Part model, mm, in its own coordinate system. Face numbers are marked on the shaded views. Give positions to 0.01 mm unless a question says otherwise; leave off trailing zeros. Order: outer loops, then holes, each group sorted by start corner. A loop starts at its lowest first (then second) coordinate and runs counter-clockwise, first axis right, second up. Notation, with made-up numbers: M 43,24 L 94,24 A33 cw 94,62 Z; hole C 55.5,49 d3. An arc over 180 degrees is marked long. Return JSON: item names as keys, results as strings.
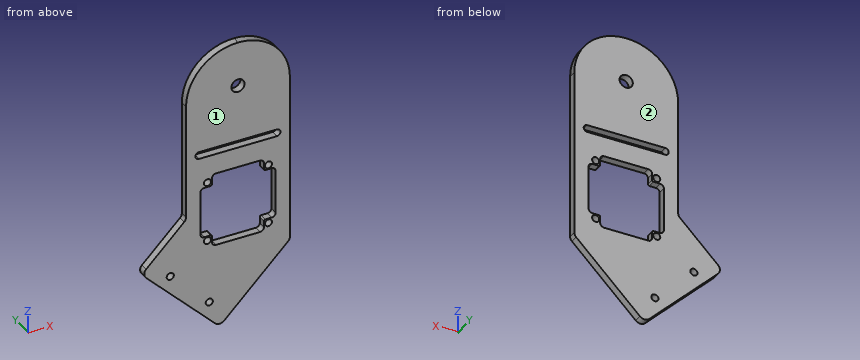
Autodesk Inventor part; units mm, degrees
ref_plane "Work Plane1" through (-29.9987, 0, 7.4992) normal (0, 0, 1) x (1, 0, 0)
ref_plane "YZ Plane" through (0, 0, 0) normal (1, 0, 0) x (0, 1, 0)
ref_plane "XZ Plane" through (0, 0, 0) normal (0, 1, 0) x (-1, 0, 0)
sketch "Sketch1" plane through (0, 0, 0) normal (0, 1, 0) x (-1, 0, 0)
  line L0 (40, 90) -> (-40, 90)
  line L1 (-40, 90) -> (-40, -81.7795)
  line L2 (40, -41.5685) -> (40, 90)
  line L3 (40, 90) -> (-40, -90) construction
  line L4 (-40, 90) -> (40, -90) construction
  circle A0 centre (-0.0013, 54.9992) radius 5.1
  line L5 (23.4987, -16.5008) -> (-23.5013, -16.5008) construction
  line L6 (-23.5013, -16.5008) -> (-23.5013, -63.5008) construction
  line L7 (-23.5013, -63.5008) -> (23.4987, -63.5008) construction
  line L8 (23.4987, -63.5008) -> (23.4987, -16.5008) construction
  line L9 (23.4987, -16.5008) -> (-23.5013, -63.5008) construction
  line L10 (-23.5013, -16.5008) -> (23.4987, -63.5008) construction
  circle A1 centre (23.4987, -16.5008) radius 2.75
  circle A2 centre (23.4987, -63.5008) radius 2.75
  circle A3 centre (-23.5013, -16.5008) radius 2.75
  circle A4 centre (-23.5013, -63.5008) radius 2.75
  line L11 (-0.0013, -90.0008) -> (-0.0013, -80) construction
  line L12 (19.9987, -11.0008) -> (-20.0013, -11.0008)
  line L13 (-20.0013, -11.0008) -> (-20.0013, -69.0008)
  line L14 (-20.0013, -69.0008) -> (19.9987, -69.0008)
  line L15 (19.9987, -69.0008) -> (19.9987, -11.0008)
  line L16 (19.9987, -11.0008) -> (-20.0013, -69.0008) construction
  line L17 (-20.0013, -11.0008) -> (19.9987, -69.0008) construction
  line L18 (-29.0013, -60.0008) -> (28.9987, -60.0008)
  line L19 (28.9987, -60.0008) -> (28.9987, -20.0008)
  line L20 (28.9987, -20.0008) -> (-29.0013, -20.0008)
  line L21 (-29.0013, -20.0008) -> (-29.0013, -60.0008)
  line L22 (-29.0013, -60.0008) -> (28.9987, -20.0008) construction
  line L23 (28.9987, -60.0008) -> (-29.0013, -20.0008) construction
  line L24 (-0.0013, 54.9992) -> (102.5291, -47.5313) construction
  line L25 (-0.0013, 54.9992) -> (144.9987, 54.9992) construction
  line L26 (28.2843, 83.2843) -> (-28.2843, 26.7157) construction
  line L27 (-28.2843, 26.7157) -> (74.2462, -75.8148) construction
  line L28 (74.2462, -75.8148) -> (130.8148, -19.2462) construction
  line L29 (130.8148, -19.2462) -> (28.2843, 83.2843) construction
  line L30 (28.2843, 83.2843) -> (74.2462, -75.8148) construction
  line L31 (-28.2843, 26.7157) -> (130.8148, -19.2462) construction
  line L32 (74.2462, -75.8148) -> (14.1407, -135.9202)
  line L33 (14.1407, -135.9202) -> (-0.0014, -121.7781)
  line L34 (-0.0014, -121.7781) -> (-31.7795, -90)
  line L35 (74.2462, -75.8148) -> (40, -41.5685)
  line L36 (-31.7795, -90) -> (-40, -81.7795)
  line L37 (44.1935, -105.8675) -> (37.1224, -98.7964)
  line L38 (37.1224, -98.7964) -> (52.1488, -83.7701) construction
  line L39 (37.1224, -98.7964) -> (22.096, -113.8228) construction
  circle A5 centre (52.1488, -83.7701) radius 2.75
  circle A6 centre (22.096, -113.8228) radius 2.75
  line L40 (-0.0013, 54.9992) -> (-0.0013, -40.0008)
  point P0 (0, 0)
  point P1 (51.2639, 3.7339)
  point P2 (-0.0013, -40.0008)
  dimension "d0" = 80
  dimension "d1" = 180
  dimension "d3" = 10.2
  dimension "d5" = 47
  dimension "d6" = 47
  dimension "d7" = 5.5
  dimension "d8" = 5.5
  dimension "d9" = 5.5
  dimension "d10" = 5.5
  dimension "d12" = 40
  dimension "d13" = 58
  dimension "d14" = 58
  dimension "d15" = 40
  dimension "d27" = 45
  dimension "d28" = 145
  dimension "d29" = 80
  dimension "d30" = 145
  dimension "d31" = 85.002
  dimension "d32" = 20
  dimension "d33" = 10
  dimension "d35" = 21.2505
  dimension "d36" = 21.2505
  dimension "d37" = 5.5
  dimension "d38" = 5.5
  dimension "d53" = 95
extrude "Plate3" add sketch "Sketch1" along normal blind 6
fillet "Fillet6" radius 5 4 edges at (-40, 3, -41.5685) (-74.2462, 3, -75.8148) (-14.1407, 3, -135.9202) (40, 3, -81.7795)
fillet "Fillet7" radius 40 2 edges at (40, 3, 90) (-40, 3, 90)
sketch "Sketch2" plane through (0, 0, 0) normal (0, -1, 0) x (1, 0, 0)
  circle A0 centre (0.0013, 54.9992) radius 5.1
  line L0 (0.0013, 54.9992) -> (0.0013, -40.0008) construction
  line L1 (0.0013, 7.4992) -> (55.0013, 7.4992) construction
  line L2 (0.0013, 7.4992) -> (-54.9987, 7.4992) construction
  line L3 (-29.9987, 7.4992) -> (30.0013, 7.4992) construction
  line L4 (-29.9987, 4.7492) -> (30.0013, 4.7492)
  line L5 (30.0013, 10.2492) -> (-29.9987, 10.2492)
  arc A1 (-29.9987, 10.2492) -> (-29.9987, 4.7492) centre (-29.9987, 7.4992) ccw
  arc A2 (30.0013, 4.7492) -> (30.0013, 10.2492) centre (30.0013, 7.4992) ccw
  point P0 (0, 0)
  dimension "d43" = 95
  dimension "d44" = 55
  dimension "d45" = 55
  dimension "d46" = 30
  dimension "d47" = 5.5
extrude "Extrusion1" cut sketch "Sketch2" against normal blind 10 contours A1 L5 A2 L4
fillet "Fillet9" radius 3 8 edges at (20.0013, 3, -11.0008) (29.0013, 3, -20.0008) (-28.9987, 3, -20.0008) (-19.9987, 3, -11.0008) (29.0013, 3, -60.0008) (20.0013, 3, -69.0008) (-28.9987, 3, -60.0008) (-19.9987, 3, -69.0008)
fillet "Fillet10" radius 1 4 edges at (-19.9987, 3, -20.0008) (20.0013, 3, -20.0008) (20.0013, 3, -60.0008) (-19.9987, 3, -60.0008)
ref_plane "Work Plane1" through (-29.9987, 0, 7.4992) normal (0, 0, 1) x (1, 0, 0)
equation "\"d39\" = Thickness"
equation "\"BendRadius\" = Thickness"
equation "\"BendReliefWidth\" = Thickness"
equation "\"BendReliefDepth\" = 0.5 * Thickness"
equation "\"CornerReliefSize\" = 4 * Thickness"
equation "\"MinimumRemnant\" = 2 * Thickness"
equation "\"TransitionRadius\" = BendRadius"
equation "\"JacobiRadiusSize\" = BendRadius"
equation "\"GapSize\" = Thickness"
properties part number "NEMA23MountPlatev2" material "Aluminum 6061"
Q1. Band-saw the part on A-A (z = -26.5). Give the cut face in (x, y), then the cut area to 3 significant figures.
Established:
{"outline": "M -40,0 L -29,0 L -29,6 L -40,6 Z; M 29,0 L 40,0 L 40,6 L 29,6 Z", "area": "132 mm²"}
Q2. Band-saw the part on D-D (z = -101.5). Give the cut face in (x, y), then the cut area to 3 significant figures.
Established:
{"outline": "M -48.56,0 L 20.28,0 L 20.28,6 L -48.56,6 Z", "area": "413 mm²"}
Q3. Pin check, flat tips, straight feed: pin 1 (2.5 mm diameter, centred on x = 23.5, y = 3.5, fed in from -Z); pin 2 (9 mm diameter, centred on x = -23.5, z = -16.5, fed in from -Y); pin 3 (1 mm diameter, centred on y = 4, z = -5, fed in from -X); pin 4 (4.5 mm diameter, centred on x = 23.5, z = -63.5, fed in from -Y). Stop position of each tip, or through.
Established:
{"pin 1": "stops at z = -99.53", "pin 2": "stops at y = 0", "pin 3": "stops at x = -40", "pin 4": "passes through"}
Q4. Band-saw the part on C-C (y = 3.5). Give the number of separate pieces and of enclosed holes in the cut face, then the cut area to 3 significant figures.
Established:
{"separate pieces": "1", "enclosed holes": "9", "area": "13,100 mm²"}
Q5. Two-plate mould, pull along Y, no slides. Class the marked faces 1 and 2: +Y half, -Y half, draft (parallel to the pull), parting line (faces both ways), or undercut.
Established:
{"face 1": "-Y half", "face 2": "+Y half"}
Q6. Probe line 1 along Z through (x, y) = (0, 4.6); line 2 along Z through (x, y) = (4.5, 0.8); line 3 along Z through (x, y) = (-25, 1.15). List the from-to ranges inside material, lowest first.
Established:
{"line 1": "z = -121.78 to -69, -11 to 4.75, 10.25 to 49.9, 60.1 to 90", "line 2": "z = -117.28 to -69, -11 to 4.75, 10.25 to 52.6, 57.4 to 89.75", "line 3": "z = -125.06 to -65.8, -61.2 to -60, -20 to -18.8, -14.2 to 4.75, 10.25 to 81.23"}
Q7. Band-saw the part on B-B (x = 13). Give the cut face in (y, z).
Established:
{"outline": "M 0,-108.78 L 6,-108.78 L 6,-69 L 0,-69 Z; M 0,-11 L 6,-11 L 6,4.75 L 0,4.75 Z; M 0,10.25 L 6,10.25 L 6,87.83 L 0,87.83 Z"}
